CAD build for the part. Positions are in the model's coordinates, mm. A direction names the side the tool comes from. Coordinates: 2 decimals unless noted, no trailing zeros. Order: outer loops, then holes, each group sorted by start corner. A loop starts at its lowest first (then second) coordinate and runs counter-clockwise, first axis right, second up.
from build123d import *

# Parameters (mm, degrees)
SKETCH_1_W               = 12
SKETCH_1_H               = 12
EXTRUDE_1_DEPTH          = 30
SKETCH_2_R               = 1.5
EXTRUDE_2_DEPTH          = 10
FILLET_1_R               = 0.5
CUT_EXTRUDE_1_DEPTH      = 1
CUT_EXTRUDE_1_DEPTH_BACK = 9
SKETCH_4_R               = 1.5
EXTRUDE_3_DEPTH          = 10
CUT_EXTRUDE_3_DEPTH      = 1
CUT_EXTRUDE_3_DEPTH_BACK = 9


with BuildPart() as part:
    # 草图1 → 凸台-拉伸1 (new body)
    with BuildSketch(Plane.XY):
        Rectangle(SKETCH_1_W, SKETCH_1_H)
    extrude(amount=EXTRUDE_1_DEPTH)

    # 草图2 → 凸台-拉伸2 (add)
    with BuildSketch(Plane.XY.offset(30)):
        Circle(SKETCH_2_R)
    extrude(amount=EXTRUDE_2_DEPTH)

    # 圆角1
    fillet_1_edges = [part.edges().sort_by_distance(p)[0] for p in [
        (-6, 0, 30),
        (0, -6, 30),
        (6, 0, 30),
        (0, -6, 0),
        (-6, 0, 0),
        (0, 6, 0),
        (6, 0, 0),
        (6, -6, 15),
        (-6, -6, 15),
        (-6, 6, 15),
        (6, 6, 15),
        (0, 6, 30),
    ]]
    fillet(fillet_1_edges, radius=FILLET_1_R)

    # 草图3 → 切除-拉伸1 (cut, two sides)
    with BuildSketch(Plane.XY.offset(40)) as cut_extrude_1_sk:
        Polygon((-31.084646908, 1), (-1.118033989, 1), (1.118033989, 1), (31.084646908, 1), (31.084646908, 60.933225838), (-31.084646908, 60.933225838), align=None)
    extrude(amount=CUT_EXTRUDE_1_DEPTH, mode=Mode.SUBTRACT)
    extrude(cut_extrude_1_sk.sketch, amount=-CUT_EXTRUDE_1_DEPTH_BACK, mode=Mode.SUBTRACT)

    # 草图4 → 凸台-拉伸3 (add)
    with BuildSketch(Plane(origin=(0, 0, 0), x_dir=(-1, 0, 0), z_dir=(0, 0, -1))):
        Circle(SKETCH_4_R)
    extrude(amount=EXTRUDE_3_DEPTH)

    # 草图5 → 切除-拉伸3 (cut, two sides)
    with BuildSketch(Plane(origin=(0, 0, -10), x_dir=(-1, 0, 0), z_dir=(0, 0, -1))) as cut_extrude_3_sk:
        Polygon((31.084646908, 1), (1.118033989, 1), (-1.118033989, 1), (-31.084646908, 1), (-31.084646908, 60.933225838), (31.084646908, 60.933225838), align=None)
    extrude(amount=CUT_EXTRUDE_3_DEPTH, mode=Mode.SUBTRACT)
    extrude(cut_extrude_3_sk.sketch, amount=-CUT_EXTRUDE_3_DEPTH_BACK, mode=Mode.SUBTRACT)


solid = part.part
1) Drill centre lines: probe 1 along Z at (x, y) = (-1, 2); probe 2 along Z at (x, y) = (0.5, 5.75); probe 3 along Y at (x, z) = (-1.25, 33). Where is each one in solid material? Low to high.
2) Pin check, flat tips, straight feed: P1, Ø0.7, axis at x = 0, z = 36.5, coming from the +Y side; P2, Ø1, axis at x = 2.5, y = -2, coming from the -Z side; P3, Ø3, axis at x = -4, y = 4, coming from the +Z side. Stop position of each tip, or through.
3) Slice it at A-A (y = -1). List the corners of the cut face in (x, z), plus the area to 3 significant figures.
4) Which spindle directions (+Z, -Z, +X, -X, +Y, -Y) get a long thin tool onto all of the face, cutting with end or side? Do faces 1 (the flat face through (-1.3, 1.3, 30)), 2 (the flat face through (0, 1, -6)), 3 (the cylindrical face through (0.325, -1.464, -4.93)), 4 (the flat face through (0, 1, 36)). Say none if no direction does.
5) Slice it at B-B (x = 0). List the corners of the cut face in (y, z).
Worked out:
1. probe 1: z = 0 to 30
1. probe 2: z = 0.07 to 29.93
1. probe 3: y = -0.83 to 0.83
2. P1: stops at y = 1
2. P2: stops at z = 0
2. P3: stops at z = 30
3. outline: (-6, 0.5) arc R0.5 ccw to (-5.5, 0) - (-1.12, 0) - (-1.12, -10) - (1.12, -10) - (1.12, 0) - (5.5, 0) arc R0.5 ccw to (6, 0.5) - (6, 29.5) arc R0.5 ccw to (5.5, 30) - (1.12, 30) - (1.12, 40) - (-1.12, 40) - (-1.12, 30) - (-5.5, 30) arc R0.5 ccw to (-6, 29.5) - close
3. area: 405 mm2
4. face 1: +Z
4. face 2: -Z, +X, -X, +Y
4. face 3: -Z
4. face 4: +Z, +X, -X, +Y
5. outline: (-6, 0.5) arc R0.5 ccw to (-5.5, 0) - (-1.5, 0) - (-1.5, -10) - (1, -10) - (1, -1) - (1.5, -1) - (1.5, 0) - (5.5, 0) arc R0.5 ccw to (6, 0.5) - (6, 29.5) arc R0.5 ccw to (5.5, 30) - (1.5, 30) - (1.5, 31) - (1, 31) - (1, 40) - (-1.5, 40) - (-1.5, 30) - (-5.5, 30) arc R0.5 ccw to (-6, 29.5) - close
